Input: part model. Units: mm. Frame: model coordinates. A direction names the side the tool comes from. Give positions to 0.01 mm unless a question says otherwise; leave off trailing zeros. Loops run counter-clockwise (first coordinate to the right, second up) from the corner with the lowest first, then second, coordinate; pieces in that order, holes last. Notation, with made-up numbers: (81, 4) -> (129, 4) arc R21 ccw to (129, 16) -> close; hole circle Ø2 at (44, 32). An arc over 180 degrees is marked (long way). Answer in a Markdown table with one row per item. Add a question column.
```python
from build123d import *

# Parameters (mm, degrees)
ESQUISSE1_R        = 10
BOSS_EXTRU_1_DEPTH = 20


with BuildPart() as part:
    # Esquisse1 → Boss.-Extru.1 (new body)
    with BuildSketch(Plane.XY):
        with BuildLine():
            Line((-1.861405692, 29.942197128), (-117.403809643, 96.650635152))
            ThreePointArc((-117.403809643, 96.650635152), (-151.55444502, 87.500001112), (-142.40381098, 53.349365735))
            Line((-142.40381098, 53.349365735), (-26.861407029, -13.359072289))
            ThreePointArc((-26.861407029, -13.359072289), (-23.344702971, -18.842102939), (-18.727404267, -23.436815684))
            Line((-18.727404267, -23.436815684), (-26.397114317, -36.72114317))
            Line((-26.397114317, -36.72114317), (-18.602885683, -41.22114317))
            Line((-18.602885683, -41.22114317), (-10.933175633, -27.936815684))
            ThreePointArc((-10.933175633, -27.936815684), (29.638157143, -4.645389236), (-1.861405692, 29.942197128))
        make_face()
        with Locations((-129.903810312, 75.000000443)):
            Circle(ESQUISSE1_R, mode=Mode.SUBTRACT)
        Circle(ESQUISSE1_R, mode=Mode.SUBTRACT)
    extrude(amount=BOSS_EXTRU_1_DEPTH)


solid = part.part
```
1) Section D-D on x = -16.5. Output: boundary loops of the cut face in (y, z).
2) Reachability of faces 1 (the face through (-23.402, -18.771, 9.86)), 2 (the face through (-22.55, -38.94, 9.86)) from +Z, -Z, +X, -X, +Y, -Y: full face, straight path, thin tool, end or side. Return the list, or none.
3) Pin query (flat end, axial travel): pin 1 (10 mm diameter, centred on y = 20.5, z = 12, fed in from -X); pin 2 (8 mm diameter, centred on y = 57.5, z = 10.5, fed in from +X); pin 3 (3 mm diameter, centred on x = -48.5, z = 13.5, fed in from +Y) (3 decimals); pin 4 (5 mm diameter, centred on y = 77, z = 6, fed in from -X). Return the tip coordinate at first contact, or that it passes through.
4) Section B-B on z = 14. Output: boundary loops of the cut face in (x, y).
5) Section C-C on x = -132. Output: boundary loops of the cut face in (y, z), and give its area (3 significant figures).
6) Material intervals for line 1 along Y through (x, z) = (0, 8.75); line 2 along Y through (x, z) = (-136, 10); line 3 along X through (y, z) = (0.5, 9.25), sorted ascending.
7) Section A-A on y = 0. Output: boundary loops of the cut face in (x, z), and give its area (3 significant figures).
Working result:
| question | item | result |
|---|---|---|
| 1 | outline | (-37.58, 0) -> (38.39, 0) -> (38.39, 20) -> (-37.58, 20) -> close |
| 2 | face 1 | +Z, -Z, -X |
| 2 | face 2 | +Z, -Z, -X, -Y |
| 3 | pin 1 | stops at x = -94.17 |
| 3 | pin 2 | stops at x = -42.66 |
| 3 | pin 3 | stops at y = 57.735 |
| 3 | pin 4 | stops at x = -154.9 |
| 4 | outline | (-142.4, 53.35) -> (-26.86, -13.36) arc R30 ccw to (-18.73, -23.44) -> (-26.4, -36.72) -> (-18.6, -41.22) -> (-10.93, -27.94) arc R30 ccw (long way) to (-1.86, 29.94) -> (-117.4, 96.65) arc R25 ccw to start; hole circle Ø20 at (-129.9, 75); hole circle Ø20 at (0, 0) |
| 5 | outline | (47.34, 0) -> (65.22, 0) -> (65.22, 20) -> (47.34, 20) -> close; (84.78, 0) -> (99.91, 0) -> (99.91, 20) -> (84.78, 20) -> close |
| 5 | area | 660 mm2 |
| 6 | line 1 | y = -30 to -10, 10 to 30 |
| 6 | line 2 | y = 49.65 to 67.07, 82.93 to 99.25 |
| 6 | line 3 | x = -50.87 to -9.99, 9.99 to 30 |
| 7 | outline | (-50, 0) -> (-10, 0) -> (-10, 20) -> (-50, 20) -> close; (10, 0) -> (30, 0) -> (30, 20) -> (10, 20) -> close |
| 7 | area | 1,200 mm2 |
